Design review of the part built by this model. Coordinates are the model's own, in mm. Coordinates: 2 decimals unless noted, no trailing zeros. Write each loop counter-clockwise with the first axis right and the second up, starting at its lowest first coordinate (ties: lowest second). Pieces come first, ordered by that corner, then holes.
```python
from build123d import *

# Parameters (mm, degrees)
SKETCH1_W           = 575
SKETCH1_H           = 120
BOSS_EXTRUDE1_DEPTH = 12.7
CHAMFER1_SIZE       = 12.7


with BuildPart() as part:
    # Sketch1 → Boss-Extrude1 (new body)
    with BuildSketch(Plane.XY):
        Rectangle(SKETCH1_W, SKETCH1_H)
    extrude(amount=BOSS_EXTRUDE1_DEPTH)

    # Chamfer1
    chamfer1_edges = [part.edges().sort_by_distance(p)[0] for p in [
        (287.5, 0, 0),
        (0, -60, 0),
        (-287.5, 0, 0),
    ]]
    chamfer(chamfer1_edges, length=CHAMFER1_SIZE - 0.0001)  # a hair under: the kernel refuses the full size


solid = part.part
```
(1) Consider section C-C (z = 2.5). Give the boundary of the cut face in (x, y), plus the area to 3 significant figures.
(2) Insertion check: pin 1 Ø3 at (y, z) = (19, 9) entering from -X. The pin has a flat end and moves straight along its axis. Give the tip position at first contact, or say it passes through.
(3) Wall thickness on line 1 (X direction, y = -2.5, z = 8.75); line 2 (Y direction, x = 263.5, z = 11.75); line 3 (X direction, y = -34, z = 9.5): over which ranges is each line inside the solid? List them lowest first.
Results:
1. outline: (-277.3, -49.8) - (277.3, -49.8) - (277.3, 60) - (-277.3, 60) - close
1. area: 60,900 mm2
2. pin 1: stops at x = -285.3
3. line 1: x = -283.55 to 283.55
3. line 2: y = -59.05 to 60
3. line 3: x = -284.3 to 284.3
